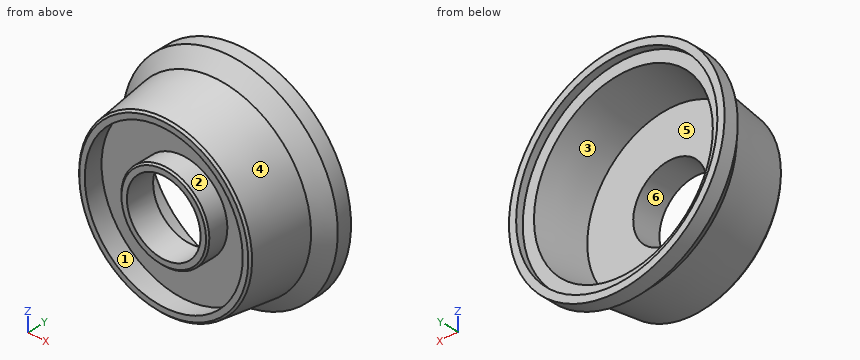
from build123d import *
from OCP.BRepFilletAPI import BRepFilletAPI_MakeChamfer

# Parameters (mm, degrees)
SHELL1_T           = -3.175
SKETCH3_R          = 16.27124
CUT_EXTRUDE1_DEPTH = 73.027519701
SHELL3_T           = -3.175
CHAMFER1_SIZE      = 0.762
CHAMFER1_SIZE2     = 0.885421272


with BuildPart() as part:
    # Sketch1 → Revolve2 (revolve)
    with BuildSketch(Plane(origin=(0, 0, 0), x_dir=(0, 0, -1), z_dir=(1, 0, 0)), mode=Mode.PRIVATE) as revolve2_sk:
        Polygon((0, 0), (38.1, 0), (42.288930477, 31.75), (47.625, 31.75), (47.625, 38.1), (0, 38.1), align=None)
    revolve(revolve2_sk.sketch.rotate(Axis((0, 0, 0), (0, -1, 0)), 180), axis=Axis((0, 0, 0), (0, -1, 0)))

    # Shell1
    shell1_openings = [part.faces().sort_by_distance(p)[0] for p in [
        (0, 38.1, 0),
    ]]
    offset(amount=SHELL1_T, openings=shell1_openings, kind=Kind.INTERSECTION)

    # Sketch2 → Revolve3 (revolve)
    with BuildSketch(Plane.XY, mode=Mode.PRIVATE) as revolve3_sk:
        Polygon((-37.277313556, 12.571930266), (0, 12.571930266), (0, 1.888797723), (-36.368110787, 1.888797723), align=None)
    revolve(revolve3_sk.sketch.rotate(Axis((0, 0, 0), (0, -1, 0)), 270), axis=Axis((0, 0, 0), (0, -1, 0)))

    # Sketch3 → Cut-Extrude1 (cut, through all)
    with BuildSketch(Plane(origin=(0, 12.571930266, 0), x_dir=(1, 0, 0), z_dir=(0, 1, 0))):
        with Locations(Location((0, 0, 0), (0, 0, 270))):
            Circle(SKETCH3_R)
    extrude(amount=-CUT_EXTRUDE1_DEPTH, mode=Mode.SUBTRACT)

    # Shell3
    shell3_openings = [part.faces().sort_by_distance(p)[0] for p in [
        (0, 0, -37.022369265),
    ]]
    offset(amount=SHELL3_T, openings=shell3_openings, kind=Kind.INTERSECTION)

    # Sketch4 → Revolve4 (revolve)
    with BuildSketch(Plane.XY, mode=Mode.PRIVATE) as revolve4_sk:
        Polygon((-47.625, 31.75), (-40.729010951, 24.854010951), (-40.729010951, 32.355083401), (-47.625, 32.355083401), align=None)
    revolve(revolve4_sk.sketch.rotate(Axis((0, 0, 0), (0, 1, 0)), 90), axis=Axis((0, 0, 0), (0, 1, 0)))

    # Chamfer1: one chamfer whose edges measure the first distance from different faces: ONE call of the kernel's chamfer builder (chamfer() names one face for all edges)
    chamfer1_edges_1 = [part.edges().sort_by_distance(p)[0] for p in [
        (0, 0, -19.44624),
    ]]
    chamfer1_edges_2 = [part.edges().sort_by_distance(p)[0] for p in [
        (0, 0, -38.1),
    ]]
    chamfer1_side_2 = [part.faces().sort_by_distance(p)[0] for p in [
        (0, 0, -35.975116662),
    ]]
    chamfer1 = BRepFilletAPI_MakeChamfer(part.part.solid().wrapped)
    for e in chamfer1_edges_1:
        chamfer1.Add(CHAMFER1_SIZE, e.wrapped)
    for e in chamfer1_edges_2:
        chamfer1.Add(CHAMFER1_SIZE, CHAMFER1_SIZE2, e.wrapped, chamfer1_side_2[0].wrapped)  # the first distance lies on this face
    add(Compound.cast(chamfer1.Shape()), mode=Mode.REPLACE)


solid = part.part
Input: part model. Units: mm. Frame: model coordinates. Face numbers are marked on the shaded views. A direction names the side the tool comes from. Round coordinates to 2 decimals unless told otherwise and drop trailing zeros. Loops run counter-clockwise (first coordinate to the right, second up) from the corner with the lowest first, then second, coordinate; pieces in that order, holes last. Notation, with made-up numbers: (49, 5.5) -> (101, 5.5) arc R13 ccw to (101, 24.5) -> close; hole circle Ø1 at (-39.75, -2). An arc over 180 degrees is marked (long way). Answer as a JSON object with one key per item and string values. Group by question number.
1) Draft query along Y for the marked faces 1, 2, 3 and 4. Return one class per face: +Y half, -Y half, draft (parallel to the pull), parting line (faces both ways), or undercut.
2) Ray query, L1, parallel to X at y = 36, z = 0 (3 decimals); L2, parallel to X at y = 7, z = 0; L3, parallel to X at y = 3.25, z = 0. Return the intervals inside material, ascending.
3) Section query D-D on y = 28. Output: boundary loops of the cut face in (x, z) (3 decimals).
4) Reachability of the marked faces 5 and 6 from +Z, -Z, +X, -X, +Y, -Y: full face, straight path, thin tool, end or side. Return the list, or none.
5) Pin query (flat end, axial travel): pin 1 (10 mm diameter, centred on x = -32.5, z = 6.5, fed in from -Y); pin 2 (4 mm diameter, centred on x = 1.5, z = -14.5, fed in from +Y); pin 3 (10 mm diameter, centred on y = 5, z = 19, fed in from +X); pin 4 (5 mm diameter, centred on x = 27.5, z = -10, fed in from -Y). Return the tip coordinate at first contact, or that it passes through.
6) Section query C-C on y = 6.5. Output: boundary loops of the cut face in (x, z).
Reply:
{
 "1": {"face 1": "undercut", "face 2": "draft", "face 3": "+Y half", "face 4": "-Y half"},
 "2": {"L1": "x = -47.625 to -44.45, 44.45 to 47.625", "L2": "x = -39.02 to -35.82, -19.45 to -16.27, 16.27 to 19.45, 35.82 to 39.02", "L3": "x = -38.53 to -35.33, -19.45 to -16.27, 16.27 to 19.45, 35.33 to 38.53"},
 "3": {"outline": "circle Ø87.75 at (0, 0); hole circle Ø77.183 at (0, 0)"},
 "4": {"face 5": "+Y", "face 6": "+Y, -Y"},
 "5": {"pin 1": "stops at y = 0", "pin 2": "stops at y = 12.57", "pin 3": "stops at x = 36.27", "pin 4": "stops at y = 9.4"},
 "6": {"outline": "circle Ø77.92 at (0, 0); circle Ø38.89 at (0, 0); hole circle Ø71.51 at (0, 0); hole circle Ø32.54 at (0, 0)"}
}
